Part print with two shaded views. Sizes in mm from the minimum x, y, z corner. Coordinates: 2 decimals unless noted, no trailing zeros. Loops run counter-clockwise (first coordinate to the right, second up) from the corner with the lowest first, then second, coordinate; pieces in that order, holes last. Notation, with made-up numbers: (64.25, 69.25) -> (81.25, 69.25) arc R10 ccw to (81.25, 78.25) -> close; hole circle Ø5 at (0.5, 35.25). An arc over 180 degrees is marked (long way). Use one line per item in the form item = value.
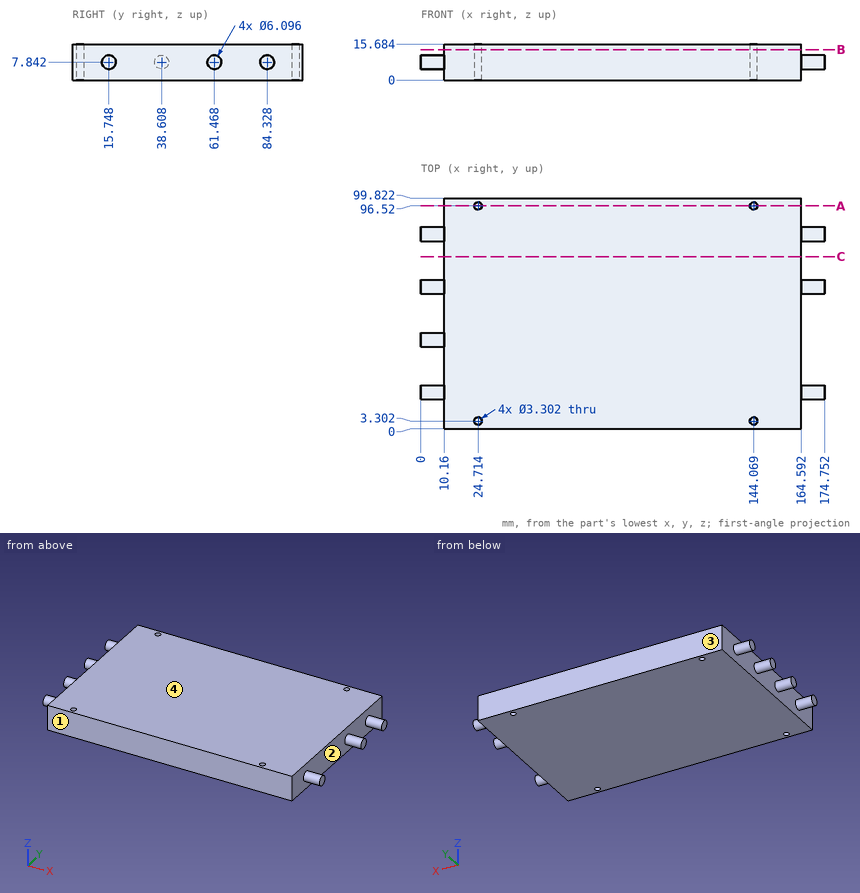
Q1. Mould opens along Y. For the marked faces 1, 2, 3 and 4 say: released by +Y, released by -Y, zero draft, split by the parting line, or undercut.
Result:
face_1 = released by -Y
face_2 = undercut
face_3 = released by +Y
face_4 = zero draft
Q2. Band-saw the part on A-A, the plane y = 96.52. Write the cut outline in (x, z) (1 decimal), and give its area (3 significant figures).
Result:
outline = (10.2, 0) -> (23.1, 0) -> (23.1, 15.7) -> (10.2, 15.7) -> close; (26.4, 0) -> (142.4, 0) -> (142.4, 15.7) -> (26.4, 15.7) -> close; (145.7, 0) -> (164.6, 0) -> (164.6, 15.7) -> (145.7, 15.7) -> close
area = 2,320 mm2
Q3. Pin check, flat tips, straight feed: pin 1 Ø8 at (y, z) = (77, 7.5) entering from +X; pin 2 Ø3 at (x, y) = (24.71, 96.52) entering from +Z; pin 3 Ø2 at (y, z) = (10.5, 7) entering from -X. Stop position of each tip, or through.
Result:
pin_1 = 164.59
pin_2 = through
pin_3 = 10.16
Q4. Wall check: line 1 along Y through (x, z) = (145.5, 4.25) (1 decimal); line 2 along X through (y, z) = (34, 2). Give the ranges that are in metal, low to high.
Result:
line_1 = 0 to 2.5, 4.1 to 95.7, 97.3 to 99.8
line_2 = 10.16 to 164.59
Q5. Band-saw the part on B-B, the plane z = 13.25. State how many separate pieces and enclosed holes the cut face has, and give its area (3 significant figures).
Result:
separate_pieces = 1
enclosed_holes = 4
area = 15,400 mm2
Q6. Band-saw the part on C-C, the plane y = 74.5. Write the cut outline in (x, z) (1 decimal).
Result:
outline = (10.2, 0) -> (164.6, 0) -> (164.6, 15.7) -> (10.2, 15.7) -> close
